Source: CAD feature listing. Evaluate the final solid. Frame: model axes, mm. A direction names the side the tool comes from. Coordinates: 2 decimals unless noted, no trailing zeros. Loops run counter-clockwise (first coordinate to the right, second up) from the corner with the lowest first, then second, coordinate; pieces in that order, holes last. Notation, with made-up numbers: M -34,-35.5 L -20,-35.5 A27 ccw -20,-16.5 Z; hole C -6.75,24.5 d5. An arc over 180 degrees is marked long. Write each question's results on one line, items separated by ' | '. Start each with the question number.
from build123d import *

# Parameters (mm, degrees)
SKETCH1_W           = 31.5468
SKETCH1_H           = 7.62
SKETCH1_R           = 0.7239
SKETCH1_W_2         = 1.5875
SKETCH1_H_2         = 1.27
BOSS_EXTRUDE1_DEPTH = 1.5875


with BuildPart() as part:
    # Sketch1 → Boss-Extrude1 (new body)
    with BuildSketch(Plane.XY):
        with Locations((-2.2606, 0)):
            Rectangle(SKETCH1_W, SKETCH1_H)
        with Locations((-15.0876, 0)):
            Circle(SKETCH1_R, mode=Mode.SUBTRACT)
        with Locations(Location((10.5664, 0, 0), (0, 0, 180))):
            Circle(SKETCH1_R, mode=Mode.SUBTRACT)
        with Locations((-16.66875, 0.635)):
            Rectangle(SKETCH1_W_2, SKETCH1_H_2, mode=Mode.SUBTRACT)
        with Locations((12.14755, 0.635)):
            Rectangle(SKETCH1_W_2, SKETCH1_H_2, mode=Mode.SUBTRACT)
    extrude(amount=BOSS_EXTRUDE1_DEPTH)


solid = part.part
Item 1: Mould query, pull axis X, two halves, no side actions, for faces 3 (the flat face through (-15.875, 1, 1)), 4 (the flat face through (13.513, 0, 1)), 5 (the flat face through (-2, 3.81, 1)). Classes: +X half, -X half, draft (parallel to the pull), parting line (faces both ways), or undercut.
Item 2: Line query: probe 1 along Y at (x, z) = (11.5, 1.05); probe 2 along X at (y, z) = (-0.25, 0.95); probe 3 along X at (y, z) = (-0.5, 0.6). Output: solid intervals per line, ascending.
Item 3: Cut plane A-A (z = 0.6). Output: boundary loops of the cut face in (x, y) (1 decimal).
Item 4: Access query for faces 1 (the flat face through (-2, 0, 1.588)), 2 (the flat face through (-17, 1.27, 1)). Directions: +Z, -Z, +X, -X, +Y, -Y. A direction counts if a zero-diameter tool reaches every point of the face in a straight line with its end or side. Return the directions, or none.
Response values:
1) face 3: undercut | face 4: +X half | face 5: draft
2) probe 1: y = -3.81 to 0, 1.27 to 3.81 | probe 2: x = -18.03 to -15.77, -14.41 to 9.89, 11.25 to 13.51 | probe 3: x = -18.03 to -15.61, -14.56 to 10.04, 11.09 to 13.51
3) outline: M -18,-3.8 L 13.5,-3.8 L 13.5,3.8 L -18,3.8 Z; hole M -17.5,0 L -15.9,0 L -15.9,1.3 L -17.5,1.3 Z; hole C -15.1,0 d1.4; hole C 10.6,0 d1.4; hole M 11.4,0 L 12.9,0 L 12.9,1.3 L 11.4,1.3 Z
4) face 1: +Z, +X, -X, +Y, -Y | face 2: +Z, -Z
